For this review, use the dimensioned drawing (mm, ordinates from the lowest corner) and the shaded views. A direction names the side the tool comes from. Coordinates: 2 decimals unless noted, no trailing zeros. Order: outer loops, then holes, each group sorted by start corner. A loop starts at its lowest first (then second) coordinate and runs counter-clockwise, first axis right, second up. Notation, with made-up numbers: M 39.25,88 L 43.25,88 A19 ccw 43.25,99 Z; hole C 62,9 d7. An arc over 180 degrees is marked long. One line per item, written item: value.
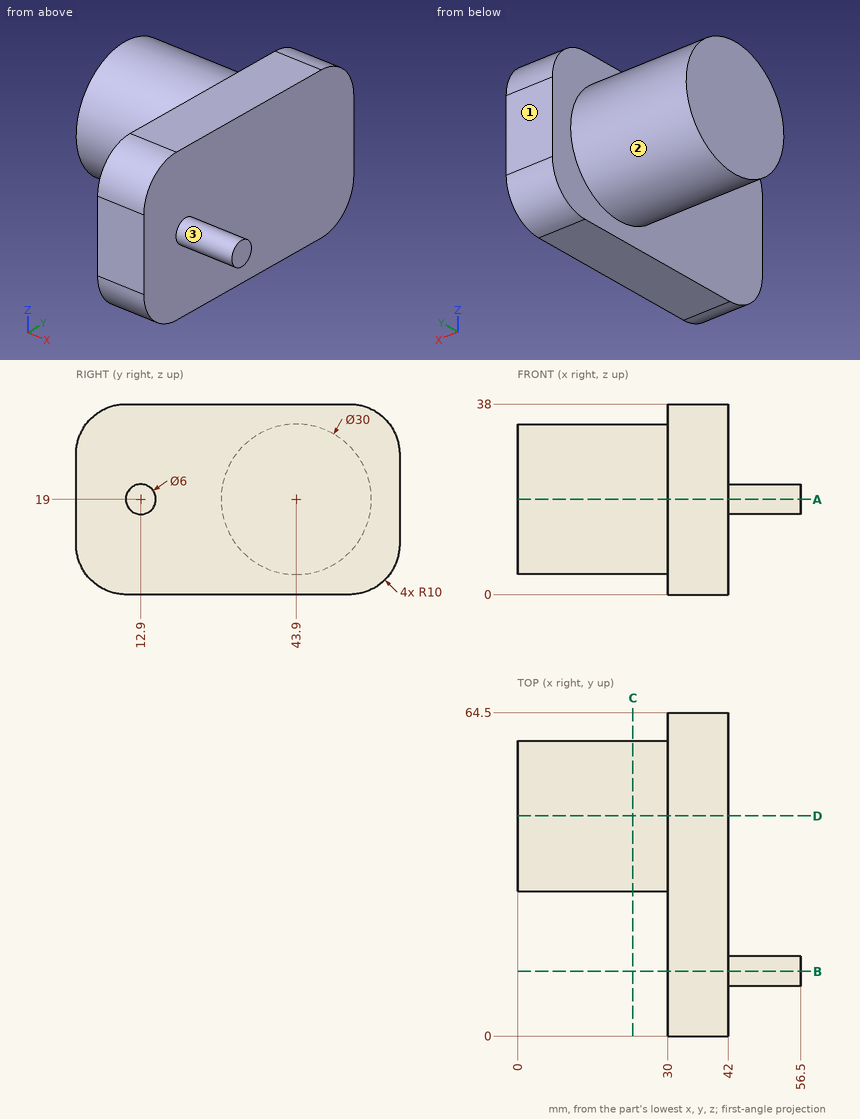
(1) We need section B-B, the plane y = 12.9. State the section outline as (x, z) points.
Geometry results:
outline: M 30,0 L 42,0 L 42,16 L 56.5,16 L 56.5,22 L 42,22 L 42,38 L 30,38 Z
(2) Tool access review of the marked faces 1, 2 and 3: name each direction out of +Z, -Z, +X, -X, +Y, -Y from which nothing blocks a thin tool from reaching the whole face with its end or side.
Geometry results:
face 1: +Z, -Z, +X, -X, +Y
face 2: -X
face 3: +X
(3) For L1, parallel to X at y = 10.5, z = 35; L2, parallel to Y at x = 13.5, z = 19.5; L3, parallel to X at y = 42, z = 29, list the stretches that pass through material, from the lowest coordinate up.
Geometry results:
L1: x = 30 to 42
L2: y = 28.91 to 58.89
L3: x = 0 to 42
(4) We need section A-A, the plane z = 19. State the section outline as (x, y) points.
Geometry results:
outline: M 0,28.9 L 30,28.9 L 30,0 L 42,0 L 42,9.9 L 56.5,9.9 L 56.5,15.9 L 42,15.9 L 42,64.5 L 30,64.5 L 30,58.9 L 0,58.9 Z
(5) We need section D-D, the plane y = 43.9. State the section outline as (x, z) points, plus the area to 3 significant figures.
Geometry results:
outline: M 0,4 L 30,4 L 30,0 L 42,0 L 42,38 L 30,38 L 30,34 L 0,34 Z
area: 1,360 mm2
(6) We need section C-C, the plane x = 23. State the section outline as (y, z) points, plus the area to 3 significant figures.
Geometry results:
outline: C 43.9,19 d30
area: 707 mm2
(7) Insertion check: pin 1 Ø4 at (y, z) = (29.5, 8.5) entering from -X; pin 2 Ø4 at (x, z) = (7, 18.5) entering from +Y; pin 3 Ø19 at (y, z) = (27, 14.5) entering from +X. Each pin has a flat end and moves straight along its axis. Give the tip position at first contact, or say it passes through.
Geometry results:
pin 1: stops at x = 30
pin 2: stops at y = 58.9
pin 3: stops at x = 42
